For this review, use the dimensioned drawing (mm, ordinates from the lowest corner) and the shaded views. A direction names the side the tool comes from. Give positions to 0.01 mm unless a question says otherwise; leave off trailing zeros. Write each loop counter-clockwise with the first axis right and the second up, starting at its lowest first coordinate (ties: lowest second). Pieces come first, ordered by that corner, then holes. Notation, with made-up numbers: (-34.5, -8) -> (-9.5, -8) arc R26 cw to (-9.5, 6) -> close; hole circle Ø8 at (49.5, 56.5). An arc over 180 degrees is marked (long way). Write each question's results on one line, items separated by ' | '. Start each with the question number.
(1) Take a section at B-B (y = 7.5). State the section outline as (x, z) points (1 decimal).
(2) To check wall thickness, follow probe 1 along Y at (x, z) = (19, 32); probe 2 along Z at (x, y) = (17, 3); probe 3 along Z at (x, y) = (17, 7.75). State the ranges of each line that lie inside material, in increasing order.
(3) Take a section at A-A (x = 17). State the section outline as (y, z) points, plus the area to 3 significant figures.
(4) Take a section at D-D (z = 31.5). State the section outline as (x, y) points.
(5) For the marked faces 1 and 2, list the 3-axis set-ups (+Z, -Z, +X, -X, +Y, -Y) from which the entire face can be reached by the end or side of a thin tool; tool diameter is ignored.
(6) Clearance check with flat-ended pins moving along their axes: pin 1 (1 mm diameter, centred on x = 12.5, y = 2.5, fed in from -Z); pin 2 (0.8 mm diameter, centred on x = 17.5, y = 3.5, fed in from +Z); pin 3 (1.5 mm diameter, centred on y = 9.5, z = 8, fed in from -X). State where each tip first meets the part, or that it passes through.
(7) Take a section at C-C (z = 3.5). State the section outline as (x, y) points.
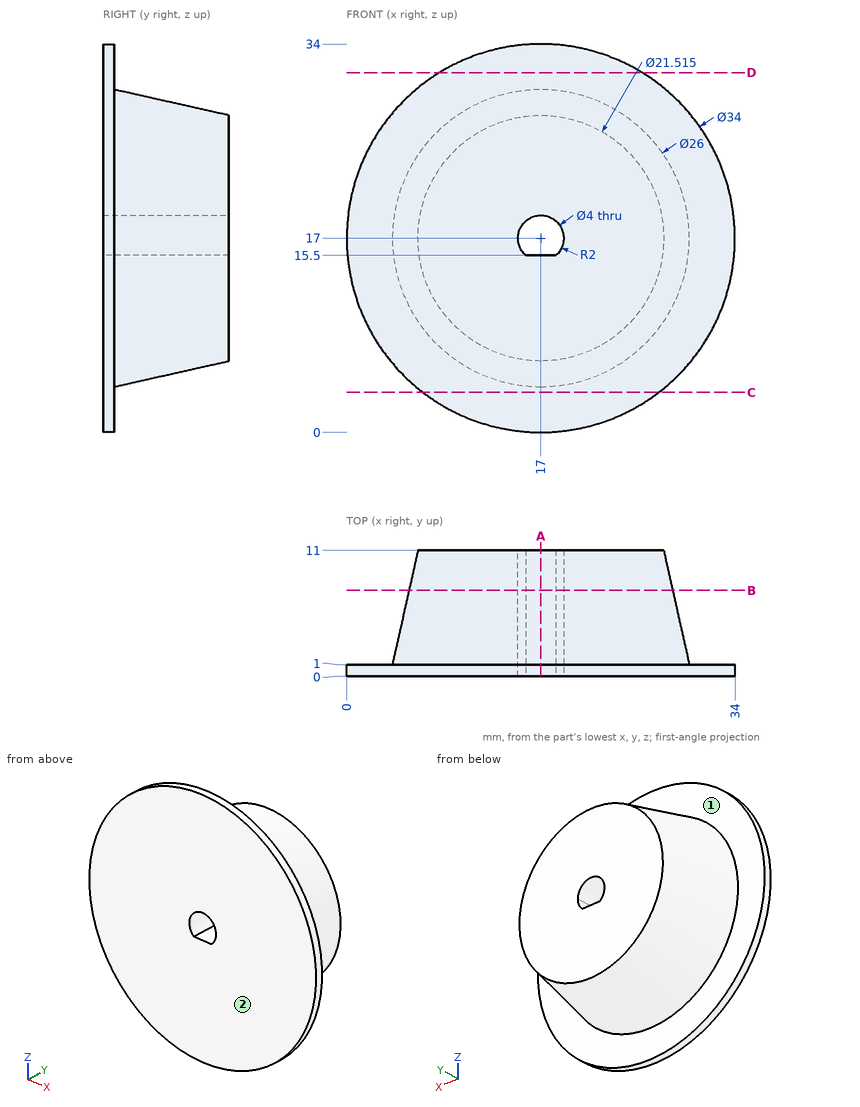
Report:
1) outline: circle Ø23.1 at (17, 17); hole (15.7, 15.5) -> (18.3, 15.5) arc R2 ccw (long way) to start
2) probe 1: 0 to 1 | probe 2: 4.45 to 15.5, 19 to 29.55 | probe 3: 5.51 to 15.5, 19 to 28.49
3) outline: (0, 0) -> (1, 0) -> (1, 4) -> (11, 6.24) -> (11, 15.5) -> (0, 15.5) -> close; (0, 19) -> (11, 19) -> (11, 27.76) -> (1, 30) -> (1, 34) -> (0, 34) -> close | area: 233 mm2
4) outline: (8.13, 0) -> (25.87, 0) -> (25.87, 1) -> (8.13, 1) -> close
5) face 1: +Y | face 2: +Z, -Z, +X, -X, -Y
6) pin 1: z = 4.95 | pin 2: z = 29.52 | pin 3: x = 9.55
7) outline: (6.67, 0) -> (27.33, 0) -> (27.33, 1) -> (6.67, 1) -> close
